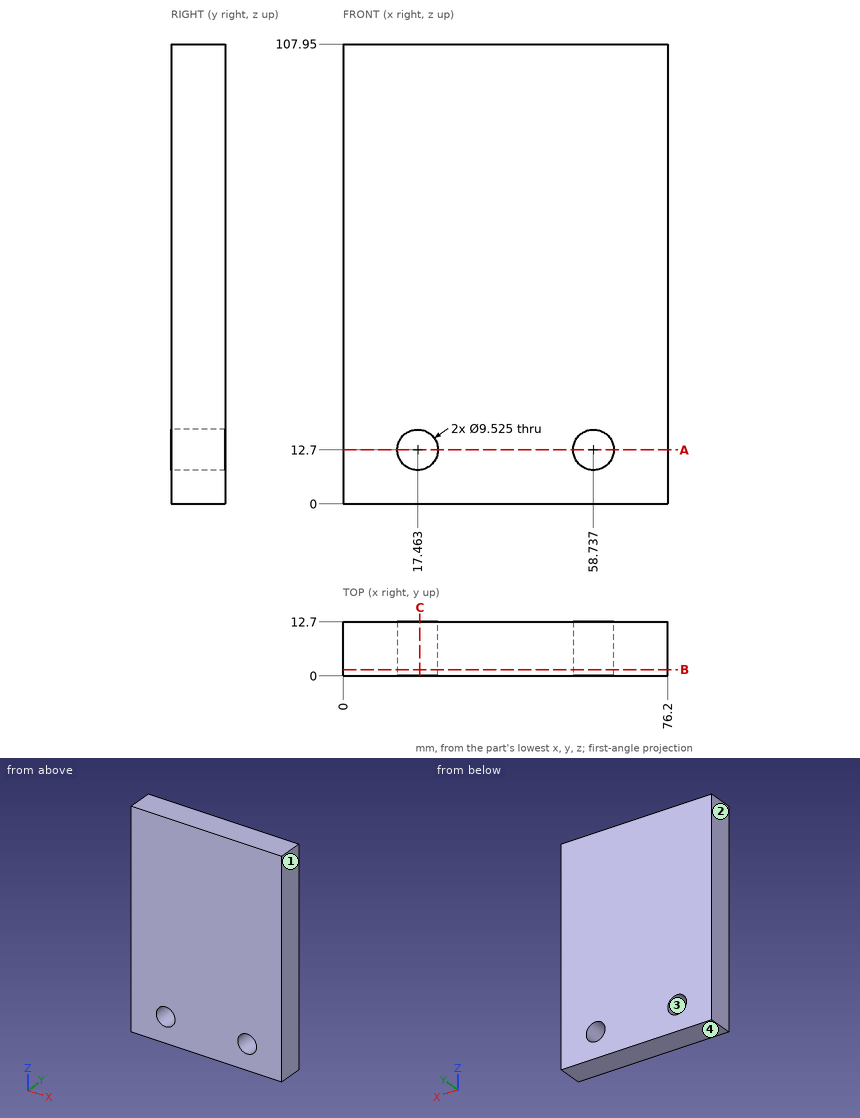
Verification items for this drawing (mm, ordinates from the low corner). Give positions to 0.01 mm unless a question says otherwise; leave off trailing zeros. Write each loop counter-clockwise with the first axis right and the second up, starting at its lowest first coordinate (ties: lowest second). Pieces come first, ordered by that corner, then holes.
1) Cross-section at C-C (x = 18). Record the boundary of the cut face in (y, z).
Values follow:
outline: (0, 0) - (12.7, 0) - (12.7, 7.97) - (0, 7.97) - close; (0, 17.43) - (12.7, 17.43) - (12.7, 107.95) - (0, 107.95) - close
2) Cross-section at A-A (z = 12.7). Record the boundary of the cut face in (x, y) (1 decimal).
Values follow:
outline: (0, 0) - (12.7, 0) - (12.7, 12.7) - (0, 12.7) - close; (22.2, 0) - (54, 0) - (54, 12.7) - (22.2, 12.7) - close; (63.5, 0) - (76.2, 0) - (76.2, 12.7) - (63.5, 12.7) - close
3) Thickness scan on line 1 (Z direction, x = 17.5, y = 4.5); line 2 (X direction, y = 6, z = 15.5) (1 decimal). Record the ranges inside material, lowest first.
Values follow:
line 1: z = 0 to 7.94, 17.46 to 107.95
line 2: x = 0 to 13.6, 21.3 to 54.9, 62.6 to 76.2
4) Release check for a two-part mould opening along X. For the marked faces 1, 2, 3 and 4 record: released by +X, released by -X, zero draft, split by the parting line, or undercut.
Values follow:
face 1: released by +X
face 2: released by -X
face 3: undercut
face 4: zero draft
5) Go/stop test with a flat-tipped pin: pin 1 Ø6 at (y, z) = (4, 95.5) entering from -X. Record where the tip stops, or that it passes through.
Values follow:
pin 1: stops at x = 0
6) Cross-section at B-B (y = 1.5). Count the separate pieces of the cut face and the enclosed holes in it, plus the area to 3 significant figures.
Values follow:
separate pieces: 1
enclosed holes: 2
area: 8,080 mm2
